Here's how the part is built. I have some questions about the finished solid (model axes, mm). Face numbers are marked on the shaded views. A direction names the side the tool comes from. Round coordinates to 2 decimals unless told otherwise and drop trailing zeros. Write each loop counter-clockwise with the first axis right and the second up, starting at its lowest first coordinate (ties: lowest second). Pieces come first, ordered by that corner, then holes. Notation, with made-up numbers: M 88,-25 L 147,-25 A18 cw 147,2 Z; hole C 72,-25 d4. An arc over 180 degrees is marked long. Use a Markdown table: item, result. Add a question column.
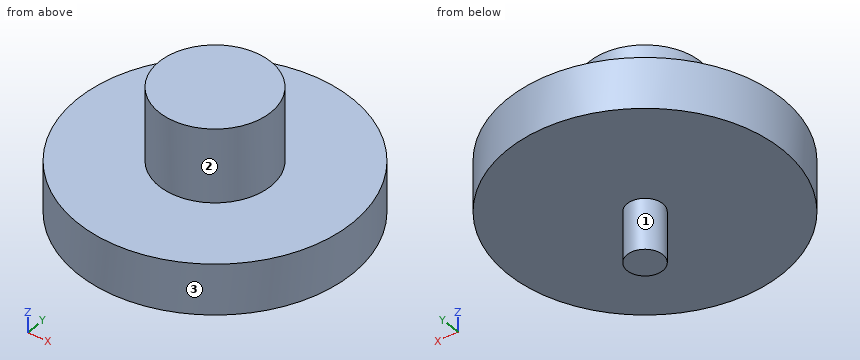
```python
from build123d import *

# Parameters (mm, degrees)
SKETCH006_R      = 54
EXTRUDE006_DEPTH = 20
SKETCH007_R      = 22
EXTRUDE007_DEPTH = 29
SKETCH008_R      = 7
EXTRUDE008_DEPTH = 20


with BuildPart() as gearholder:
    # Sketch006 (on Face123 of Fusion001) → Extrude006 (new body)
    with BuildSketch(Plane.XY.offset(10)):
        Circle(SKETCH006_R)
    extrude(amount=-EXTRUDE006_DEPTH)


with BuildPart() as motorshaftholder:
    # Sketch007 (on Face3 of Extrude006) → Extrude007 (new body)
    with BuildSketch(Plane.XY.offset(10)):
        Circle(SKETCH007_R)
    extrude(amount=EXTRUDE007_DEPTH)


with BuildPart() as obj1:
    # Sketch008 (on Face2 of Extrude006) → Extrude008 (new body)
    with BuildSketch(Plane(origin=(0, 0, -10), x_dir=(1, 0, 0), z_dir=(0, 0, -1))):
        Circle(SKETCH008_R)
    extrude(amount=EXTRUDE008_DEPTH)

    # Fusion006: union gearHolder, motorShaftHolder
    add(gearholder.part)
    add(motorshaftholder.part)


solid = obj1.part
```
Item 1: Imagine slicing it at C-C on z = 21.5. List the corners of the cut face in (x, y) for me, plus the area to 3 significant figures.
Item 2: Imagine slicing it at A-A on x = 0. List the corners of the cut face in (y, z) for me.
Item 3: On a 3-axis mill with a long thin cutter (end or side, diameter ignored), from which of +Z, -Z, +X, -X, +Y, -Y can I reach the whole of each face in a straight line? I mean the marked faces 1, 2 and 3. Say none if no direction works.
Item 4: For pin 1 Ø4 at (x, z) = (39.5, 12.5) entering from -Y (3 decimals); pin 2 Ø1.5 at (y, z) = (-25, 7) entering from -X; pin 3 Ø4 at (y, z) = (-39.5, 3.5) entering from -X; pin 4 Ø8 at (x, z) = (15, -10.5) entering from -Y, each with a flat end and sliding along its axis, tell me the tip position at first contact or that it passes through.
Item 5: I need wall thicknesses on probe 1 along Z at (x, y) = (17, -34.5); probe 2 along Z at (x, y) = (-8.5, -4); probe 3 along Y at (x, z) = (10, 16.5). Which ranges of each line are inside material? Lowest first, please. Write a range as from..to.
Item 6: Imagine slicing it at D-D on x = -16.5. List the corners of the cut face in (y, z) for me, plus the area to 3 significant figures.
The answers:
| question | item | result |
|---|---|---|
| 1 | outline | C 0,0 d44 |
| 1 | area | 1,520 mm² |
| 2 | outline | M -54,-10 L -7,-10 L -7,-30 L 7,-30 L 7,-10 L 54,-10 L 54,10 L 22,10 L 22,39 L -22,39 L -22,10 L -54,10 Z |
| 3 | face 1 | -Z |
| 3 | face 2 | +Z |
| 3 | face 3 | +Z, -Z |
| 4 | pin 1 | through |
| 4 | pin 2 | x = -48.25 |
| 4 | pin 3 | x = -38.86 |
| 4 | pin 4 | y = -52.86 |
| 5 | probe 1 | -10..10 |
| 5 | probe 2 | -10..39 |
| 5 | probe 3 | -19.6..19.6 |
| 6 | outline | M -51.42,-10 L 51.42,-10 L 51.42,10 L 14.55,10 L 14.55,39 L -14.55,39 L -14.55,10 L -51.42,10 Z |
| 6 | area | 2,900 mm² |
